from build123d import *

# Parameters (mm, degrees)
F0_R          = 57
F0_R_2        = 6
F1_DEPTH      = 16
F2_R          = 27
F3_DEPTH      = 50
F5_DEPTH      = 46.5
F6_R          = 8
F7_R          = 27
F8_DEPTH      = 44
F8_DEPTH_BACK = 25
F9_R          = 57
F9_R_2        = 27
F10_DEPTH     = 16
F11_R         = 6
F12_DEPTH     = 25
F14_DEPTH     = 37.5
F15_R         = 3
F16_R         = 3
F17_R         = 18
F18_DEPTH     = 4
F19_DEPTH     = 25
F20_R         = 27.5
F21_DEPTH     = 25


with BuildPart() as f1:
    # F0 (on Top) → F1 (new body)
    with BuildSketch(Plane.XY):
        Circle(F0_R)
        with Locations((-29.6984848098, -29.6984848098)):
            Circle(F0_R_2, mode=Mode.SUBTRACT)
        with Locations((29.6984848098, -29.6984848098)):
            Circle(F0_R_2, mode=Mode.SUBTRACT)
        with Locations((-29.6984848098, 29.6984848098)):
            Circle(F0_R_2, mode=Mode.SUBTRACT)
        with Locations((29.6984848098, 29.6984848098)):
            Circle(F0_R_2, mode=Mode.SUBTRACT)
    extrude(amount=F1_DEPTH)

    # F2 (on face) → F3 (join)
    with BuildSketch(Plane.XY.offset(16)):
        Circle(F2_R)
    extrude(amount=F3_DEPTH)

    # F4 (on Front) → F5 (join, symmetric)
    with BuildSketch(Plane.XZ):
        with BuildLine():
            Line((62, 208), (-62, 208))
            ThreePointArc((-62, 208), (-78.9705627485, 200.9705627485), (-86, 184))
            Line((-86, 184), (-86, 114))
            ThreePointArc((-86, 114), (-71.941125497, 80.058874503), (-38, 66))
            Line((-38, 66), (0, 66))
            Line((0, 66), (38, 66))
            ThreePointArc((38, 66), (71.941125497, 80.058874503), (86, 114))
            Line((86, 114), (86, 184))
            ThreePointArc((86, 184), (78.9705627485, 200.9705627485), (62, 208))
        make_face()
    extrude(amount=F5_DEPTH, both=True)

    # F6
    f6_edges = [f1.edges().sort_by_distance(p)[0] for p in [
        (0, -46.5, 208),
        (-78.970563, -46.5, 200.970563),
        (-86, -46.5, 149),
        (-71.941125, -46.5, 80.058875),
        (0, -46.5, 66),
        (71.941125, -46.5, 80.058875),
        (86, -46.5, 149),
        (78.970563, -46.5, 200.970563),
        (0, 46.5, 208),
        (-78.970563, 46.5, 200.970563),
        (-86, 46.5, 149),
        (-71.941125, 46.5, 80.058875),
        (0, 46.5, 66),
        (71.941125, 46.5, 80.058875),
        (86, 46.5, 149),
        (78.970563, 46.5, 200.970563),
    ]]
    fillet(f6_edges, radius=F6_R)

    # F7 (on face) → F8 (join, two sides)
    with BuildSketch(Plane.XY.offset(208)) as f8_sk:
        with Locations((38, 0)):
            Circle(F7_R)
    extrude(amount=F8_DEPTH)
    extrude(f8_sk.sketch, amount=-F8_DEPTH_BACK)

    # F9 (on face) → F10 (join)
    with BuildSketch(Plane.XY.offset(252)):
        with Locations((38, 0)):
            Circle(F9_R)
        with Locations((38, 0)):
            Circle(F9_R_2, mode=Mode.SUBTRACT)
        with Locations((38, 0)):
            Circle(F9_R_2)
    extrude(amount=F10_DEPTH)

    # F11 (on face) → F12 (cut)
    with BuildSketch(Plane.XY.offset(268)):
        with Locations((67.6984848098, 29.6984848098)):
            Circle(F11_R)
        with Locations((67.6984848098, -29.6984848098)):
            Circle(F11_R)
        with Locations((8.3015151902, 29.6984848098)):
            Circle(F11_R)
        with Locations((8.3015151902, -29.6984848098)):
            Circle(F11_R)
    extrude(amount=-F12_DEPTH, mode=Mode.SUBTRACT)

    # F13 (on Front) → F14 (cut, symmetric)
    with BuildSketch(Plane.XZ):
        with BuildLine():
            ThreePointArc((-77, 114), (-65.5771644663, 86.4228355337), (-38, 75))
            Line((-38, 75), (38, 75))
            ThreePointArc((38, 75), (65.5771644663, 86.4228355337), (77, 114))
            Line((77, 114), (77, 184))
            ThreePointArc((77, 184), (72.6066017178, 194.6066017178), (62, 199))
            Line((62, 199), (-62, 199))
            ThreePointArc((-62, 199), (-72.6066017178, 194.6066017178), (-77, 184))
            Line((-77, 184), (-77, 114))
        make_face()
    extrude(amount=F14_DEPTH, both=True, mode=Mode.SUBTRACT)

    # F15
    f15_edges = [f1.edges().sort_by_distance(p)[0] for p in [
        (77, 37.5, 149),
    ]]
    fillet(f15_edges, radius=F15_R)

    # F16
    f16_edges = [f1.edges().sort_by_distance(p)[0] for p in [
        (77, -37.5, 149),
    ]]
    fillet(f16_edges, radius=F16_R)

    # F17 (on face) → F18 (join)
    with BuildSketch(Plane.XZ.offset(46.5)):
        with BuildLine():
            ThreePointArc((8.4444444444, 95.2524898773), (47.7610336429, 80.3886593213), (73, 114))
            ThreePointArc((73, 114), (47.7610336429, 147.6113406787), (8.4444444444, 132.7475101227))
            ThreePointArc((8.4444444444, 132.7475101227), (3, 114), (8.4444444444, 95.2524898773))
        make_face()
        with Locations((38, 114)):
            Circle(F17_R, mode=Mode.SUBTRACT)
        with BuildLine():
            ThreePointArc((8.4444444444, 95.2524898773), (3, 114), (8.4444444444, 132.7475101227))
            ThreePointArc((8.4444444444, 132.7475101227), (0, 128.1039415864), (-8.4444444444, 132.7475101227))
            ThreePointArc((-8.4444444444, 132.7475101227), (-4.3886593213, 123.7610336429), (-3, 114))
            ThreePointArc((-3, 114), (-4.3886593213, 104.2389663571), (-8.4444444444, 95.2524898773))
            ThreePointArc((-8.4444444444, 95.2524898773), (0, 99.8960584136), (8.4444444444, 95.2524898773))
        make_face()
        with BuildLine():
            ThreePointArc((-3, 114), (-4.3886593213, 123.7610336429), (-8.4444444444, 132.7475101227))
            ThreePointArc((-8.4444444444, 132.7475101227), (-73, 114), (-8.4444444444, 95.2524898773))
            ThreePointArc((-8.4444444444, 95.2524898773), (-4.3886593213, 104.2389663571), (-3, 114))
        make_face()
        with Locations((-38, 114)):
            Circle(F17_R, mode=Mode.SUBTRACT)
    extrude(amount=F18_DEPTH)

    # F19 (cut): faces of the model
    f19_faces = [f1.faces().sort_by_distance(p)[0] for p in [
        (-38, -46.5, 114),
        (38, -46.5, 114),
    ]]
    extrude(f19_faces, amount=-F19_DEPTH, mode=Mode.SUBTRACT)

    # F20 (on face) → F21 (cut)
    with BuildSketch(Plane(origin=(0, 46.5, 0), x_dir=(-1, 0, 0), z_dir=(0, 1, 0))):
        with Locations((-38, 114)):
            Circle(F20_R)
        with Locations((38, 114)):
            Circle(F20_R)
    extrude(amount=-F21_DEPTH, mode=Mode.SUBTRACT)


solid = f1.part
Work out the finished part from the listing and answer in its coordinate system (mm). A direction names the side the tool comes from. Round coordinates to 2 decimals unless told otherwise and drop trailing zeros. Write each loop counter-clockwise with the first axis right and the second up, starting at its lowest first coordinate (ties: lowest second). Pieces come first, ordered by that corner, then holes. Notation, with made-up numbers: M 22.5,-23 L 56.5,-23 A30 ccw 56.5,4 Z; hole C 24,-2 d9. An arc over 180 degrees is marked long. Use a Markdown table: item, result.
1) The part is cut by section A-A on x = -0.5. State how many separate pieces and enclosed holes the cut face has, plus the area to 3 significant figures.
Taken from the geometry:
| item | result |
|---|---|
| separate pieces | 2 |
| enclosed holes | 1 |
| area | 9,840 mm2 |
2) Determine the mould class of faces 1 (the face through (-83.719, 44.094, 148.51)), 2 (the face through (71.57, -0.54, 79.69)) for opening direction Z: pulls with the +Z half, pulls with the -Z half, needs draft (parallel to the pull), parting line crosses it, or undercut.
Taken from the geometry:
| item | result |
|---|---|
| face 1 | needs draft |
| face 2 | undercut |
3) Consider line 1 (Z direction, x = 38, y = -47.6); line 2 (Z direction, x = 39.5, y = 27); line 3 (Z direction, x = 0.5, y = 1.5). Determine where each line is inside the solid, lowest interval first. Write a range as [from, to].
Taken from the geometry:
| item | result |
|---|---|
| line 1 | z = [79, 96], [132, 149], [252, 268] |
| line 2 | z = [0, 16], [66.02, 75.03], [199, 208], [252, 268] |
| line 3 | z = [0, 75], [199, 208], [252, 268] |
4) Flat-ended cylindrical pins translate along their axes: pin 1 (2 mm diameter, centred on y = 42, z = 106, fed in from +X); pin 2 (4 mm diameter, centred on x = -48.5, y = 21, fed in from +Z); pin 3 (21 mm diameter, centred on x = 28.5, z = 119, fed in from -Y). Find the tip coordinate at first contact, or state that the pin passes through.
Taken from the geometry:
| item | result |
|---|---|
| pin 1 | stops at x = 84.96 |
| pin 2 | stops at z = 208 |
| pin 3 | stops at y = -50.5 |
5) Which of the six approach directions +Z, -Z, +X, -X, +Y, -Y give full straight-line access (tool end or side, diameter ignored) to faces 3 (the face through (7.001, -35.556, 260.112)), 4 (the face through (-34.46, -33.35, 7.89)), 5 (the face through (-72.977, -48.472, 115.262)), 6 (the face through (-1, 37.5, 151))?
Taken from the geometry:
| item | result |
|---|---|
| face 3 | +Z |
| face 4 | -Z |
| face 5 | -Y |
| face 6 | none |
6) The part is cut by section B-B on z = 164.5. Give the vertices of the cut face in (x, y), plus the area to 3 significant figures.
Taken from the geometry:
| item | result |
|---|---|
| outline | M -86,-38.5 A8 ccw -78,-46.5 L 78,-46.5 A8 ccw 86,-38.5 L 86,38.5 A8 ccw 78,46.5 L -78,46.5 A8 ccw -86,38.5 Z; hole M -77,-34.5 A3 ccw -74,-37.5 L 74,-37.5 A3 ccw 77,-34.5 L 77,34.5 A3 ccw 74,37.5 L -74,37.5 A3 ccw -77,34.5 Z |
| area | 4,400 mm2 |
